Check sheet for the modelled part. Datum: model origin and axes. Units: mm. Round coordinates to 2 decimals unless told otherwise and drop trailing zeros. One line per item, written item: value.
from build123d import *

# Parameters (mm, degrees)
F0_R     = 2.09999979
F1_DEPTH = 400


# Not quite as in the source:
# - ends of sketch curves that miss each other by under 0.0002 mm in the source are joined


with BuildPart() as f1:
    # F0 (on Front) → F1 (new body)
    with BuildSketch(Plane.XZ):
        with BuildLine():
            Line((-4.639999536, 10), (-8.50000015, 10))
            ThreePointArc((-8.50000015, 10), (-9.5606602157, 9.5606602157), (-10, 8.50000015))
            Line((-10, 8.50000015), (-10, 4.639999536))
            Line((-10, 4.639999536), (-8.19999818, 2.839999716))
            Line((-8.19999818, 2.839999716), (-8.19999818, 5.4993384501))
            Line((-8.19999818, 5.4993384501), (-6.559999344, 5.4993384501))
            Line((-6.559999344, 5.4993384501), (-3.9006596099, 2.839999716))
            Line((-3.9006596099, 2.839999716), (-3.9006596099, 0.19999898))
            Line((-3.9006596099, 0.19999898), (-3.7006596299, -1e-06))
            Line((-3.7006596299, -1e-06), (-3.9006596099, -0.20000098))
            Line((-3.9006596099, -0.20000098), (-3.9006596099, -2.840000716))
            Line((-3.9006596099, -2.840000716), (-6.559999344, -5.4993404501))
            Line((-6.559999344, -5.4993404501), (-8.19999818, -5.4993404501))
            Line((-8.19999818, -5.4993404501), (-8.19999818, -2.840000716))
            Line((-8.19999818, -2.840000716), (-10, -4.640000536))
            Line((-10, -4.640000536), (-10, -8.50000115))
            ThreePointArc((-10, -8.50000115), (-9.5606602157, -9.5606612157), (-8.50000015, -10.000001))
            Line((-8.50000015, -10.000001), (-4.639999536, -10))
            Line((-4.639999536, -10), (-2.839999716, -8.20000018))
            Line((-2.839999716, -8.20000018), (-5.4993394501, -8.20000018))
            Line((-5.4993394501, -8.20000018), (-5.4993394501, -6.560000344))
            Line((-5.4993394501, -6.560000344), (-2.839999716, -3.9006606099))
            Line((-2.839999716, -3.9006606099), (-0.19999898, -3.9006606099))
            Line((-0.19999898, -3.9006606099), (1e-06, -3.7006606299))
            Line((1e-06, -3.7006606299), (0.20000098, -3.9006606099))
            Line((0.20000098, -3.9006606099), (2.839999716, -3.9006606099))
            Line((2.839999716, -3.9006606099), (5.4993414501, -6.560000344))
            Line((5.4993414501, -6.560000344), (5.4993414501, -8.20000018))
            Line((5.4993414501, -8.20000018), (2.839999716, -8.20000018))
            Line((2.839999716, -8.20000018), (4.639999536, -10))
            Line((4.639999536, -10), (8.50000015, -10))
            ThreePointArc((8.50000015, -10), (9.5606602157, -9.5606612157), (10, -8.50000115))
            Line((10, -8.50000115), (10, -4.640000536))
            Line((10, -4.640000536), (8.20000018, -2.840000716))
            Line((8.20000018, -2.840000716), (8.20000018, -5.4993404501))
            Line((8.20000018, -5.4993404501), (6.560000344, -5.4993404501))
            Line((6.560000344, -5.4993404501), (3.9006596099, -2.840000716))
            Line((3.9006596099, -2.840000716), (3.9006596099, -0.20000098))
            Line((3.9006596099, -0.20000098), (3.7006596299, -1e-06))
            Line((3.7006596299, -1e-06), (3.9006596099, 0.19999898))
            Line((3.9006596099, 0.19999898), (3.9006596099, 2.839999716))
            Line((3.9006596099, 2.839999716), (6.560000344, 5.4993384501))
            Line((6.560000344, 5.4993384501), (8.20000018, 5.4993384501))
            Line((8.20000018, 5.4993384501), (8.20000018, 2.839999716))
            Line((8.20000018, 2.839999716), (10, 4.639999536))
            Line((10, 4.639999536), (10, 8.50000015))
            ThreePointArc((10, 8.50000015), (9.5606602157, 9.5606602157), (8.50000015, 10))
            Line((8.50000015, 10), (4.639999536, 10))
            Line((4.639999536, 10), (2.839999716, 8.20000018))
            Line((2.839999716, 8.20000018), (5.4993414501, 8.20000018))
            Line((5.4993414501, 8.20000018), (5.4993414501, 6.559998344))
            Line((5.4993414501, 6.559998344), (2.839999716, 3.9006596099))
            Line((2.839999716, 3.9006596099), (0.20000098, 3.9006596099))
            Line((0.20000098, 3.9006596099), (1e-06, 3.7006596299))
            Line((1e-06, 3.7006596299), (-0.19999898, 3.9006596099))
            Line((-0.19999898, 3.9006596099), (-2.839999716, 3.9006596099))
            Line((-2.839999716, 3.9006596099), (-5.4993394501, 6.559998344))
            Line((-5.4993394501, 6.559998344), (-5.4993394501, 8.20000018))
            Line((-5.4993394501, 8.20000018), (-2.839999716, 8.20000018))
            Line((-2.839999716, 8.20000018), (-4.639999536, 10))
        make_face()
        Polygon((-6.5693393431, -8.20000018), (-8.19999818, -8.20000018), (-8.19999818, -6.5693403431), (-7.629998237, -6.5693403431), (-6.5693393431, -7.630000237), align=None, mode=Mode.SUBTRACT)
        Polygon((8.20000018, -8.20000018), (6.5693393431, -8.20000018), (6.5693393431, -7.630000237), (7.630002237, -6.5693403431), (8.20000018, -6.5693403431), align=None, mode=Mode.SUBTRACT)
        with Locations((1e-06, -1e-06)):
            Circle(F0_R, mode=Mode.SUBTRACT)
        Polygon((-8.19999818, 8.20000018), (-6.5693393431, 8.20000018), (-6.5693393431, 7.629999237), (-7.629998237, 6.5693393431), (-8.19999818, 6.5693393431), align=None, mode=Mode.SUBTRACT)
        Polygon((6.5693393431, 8.20000018), (8.20000018, 8.20000018), (8.20000018, 6.5693393431), (7.630002237, 6.5693393431), (6.5693393431, 7.629999237), align=None, mode=Mode.SUBTRACT)
    extrude(amount=F1_DEPTH)


solid = f1.part
Q1. Depth check by flat-ended pin: P1, Ø2, axis at y = -223.5, z = -4, coming from the -X side; P2, Ø1.5, axis at y = -249, z = -1, coming from the +X side; P3, Ø2, axis at x = 2, y = -267, coming from the +Z side; P4, Ø1, axis at y = -64, z = -2.5, coming from the -X side. Enter the tip coordinate at first touch or a pass-through.
Completed:
P1: x = -10
P2: x = 3.9
P3: z = 8.36
P4: x = -8.36
Q2. Scan lines: line 1 (Z direction, x = 8, y = -85.5); line 2 (X direction, y = -198.5, z = 8.25); line 3 (X direction, y = -204, z = 4.75). Record each from-to range of solid material in increasing order. Write a range as [from, to].
Completed:
line 1: [-10, -8.2], [-6.57, -5.5], [5.5, 6.57], [8.2, 10]
line 2: [-10, -2.89], [2.89, 10]
line 3: [-10, -8.2], [-5.81, -3.69], [3.69, 5.81], [8.2, 10]
Q3. Sectioned sample at A-A on y = -287.5. State how many separate pieces and enclosed holes the cut face has, and give its area (3 significant figures).
Completed:
separate pieces: 1
enclosed holes: 5
area: 161 mm^2
